Autodesk Inventor part; units mm, degrees
ref_plane "YZ Plane" through (0, 0, 0) normal (1, 0, 0) x (0, 1, 0)
ref_plane "XZ Plane" through (0, 0, 0) normal (0, 1, 0) x (-1, 0, 0)
ref_plane "XY Plane" through (0, 0, 0) normal (0, 0, 1) x (1, 0, 0)
sketch "Sketch1" plane through (0, 0, 0) normal (0, 0, 1) x (1, 0, 0)
  line L0 (3.175, 0) -> (3.175, 3.175)
  line L1 (3.175, 3.175) -> (-3.175, 3.175)
  line L2 (-3.175, 3.175) -> (-3.175, 0)
  line L3 (5.08, 0) -> (5.08, 5.08)
  line L4 (5.08, 5.08) -> (-5.08, 5.08)
  line L5 (-5.08, 5.08) -> (-5.08, 0)
  line L6 (-5.08, 0) -> (-3.175, 0)
  line L7 (3.175, 0) -> (5.08, 0)
  point P0 (0, 0)
  dimension "d0" = 10.16
  dimension "d1" = 5.08
extrude "Extrusion1" add sketch "Sketch1" along normal blind 139.7
sketch "Sketch2" plane through (-5.08, 5.08, 0) normal (0, 1, 0) x (1, 0, 0)
  circle A0 centre (5.08, -6.35) radius 1.985
  circle A1 centre (5.08, -133.35) radius 1.985
  circle A2 centre (5.08, -69.85) radius 1.985
  point P0 (5.08, 0)
  dimension "d4" = 3.97
  dimension "d5" = 3.97
  dimension "d10" = 3.97
extrude "Extrusion2" cut sketch "Sketch2" against normal blind 139.7
sketch "Sketch3" plane through (-5.08, 5.08, 0) normal (0, 1, 0) x (1, 0, 0)
  circle A0 centre (5.08, -6.35) radius 1.985
  circle A1 centre (5.08, -133.35) radius 1.985
  circle A2 centre (5.08, -133.35) radius 5.08
  line L0 (0, 0) -> (0, -139.7)
  circle A3 centre (5.08, -6.35) radius 5.08
  circle A4 centre (5.08, -69.85) radius 1.985
  circle A5 centre (5.08, -69.85) radius 5.08
  point P0 (5.08, 0)
extrude "Extrusion3" add sketch "Sketch3" along normal blind 6.35
properties part number "arm_xbrace_jig"
Geometry check sheet. Reference: the model listing, model coordinates, mm. A direction names the side the tool comes from. Give positions to 0.01 mm unless a question says otherwise; leave off trailing zeros. Write each loop counter-clockwise with the first axis right and the second up, starting at its lowest first coordinate (ties: lowest second). Pieces come first, ordered by that corner, then holes.
1) Release check for a two-part mould opening along Z. For faces 6 (the face through (0, 4, 0)), 7 (the face through (3.175, 2, 69)), 8 (the face through (-1.1, 8.21, 1.39)) record: released by +Z, released by -Z, zero draft, split by the parting line, or undercut.
Values follow:
face 6: released by -Z
face 7: zero draft
face 8: undercut
2) Cross-section at A-A (y = 1.25). Record the boundary of the cut face in (x, z) (3 decimals), plus the area to 3 significant figures.
Values follow:
outline: (-5.08, 0) - (-3.175, 0) - (-3.175, 139.7) - (-5.08, 139.7) - close; (3.175, 0) - (5.08, 0) - (5.08, 139.7) - (3.175, 139.7) - close
area: 532 mm2
3) Cross-section at B-B (x = 0). Record the boundary of the cut face in (y, z) (3 decimals), plus the area to 3 significant figures.
Values follow:
outline: (3.175, 0) - (5.08, 0) - (5.08, 1.27) - (11.43, 1.27) - (11.43, 4.365) - (3.175, 4.365) - close; (3.175, 8.335) - (11.43, 8.335) - (11.43, 11.43) - (5.08, 11.43) - (5.08, 64.77) - (11.43, 64.77) - (11.43, 67.865) - (3.175, 67.865) - close; (3.175, 71.835) - (11.43, 71.835) - (11.43, 74.93) - (5.08, 74.93) - (5.08, 128.27) - (11.43, 128.27) - (11.43, 131.365) - (3.175, 131.365) - close; (3.175, 135.335) - (11.43, 135.335) - (11.43, 138.43) - (5.08, 138.43) - (5.08, 139.7) - (3.175, 139.7) - close
area: 361 mm2
4) Set-up check for faces 1 (the face through (-0.258, 7.36, 4.382)), 2 (the face through (-1.1, 8.21, 64.89)), 3 (the face through (2.2, 11.43, 69.8)), 4 (the face through (0, 5.08, 1)), 5 (the face through (-2, 3.175, 69)): record each of +Z, -Z, +X, -X, +Y, -Y from which the full face is reachable in a straight line by a thin tool's end or side.
Values follow:
face 1: +Y, -Y
face 2: +Y
face 3: +Z, -Z, +X, -X, +Y
face 4: -Z, +Y
face 5: +Z, -Z, -Y
5) Cross-section at D-D (z = 116). Record the boundary of the cut face in (x, y) (3 decimals).
Values follow:
outline: (-5.08, 0) - (-3.175, 0) - (-3.175, 3.175) - (3.175, 3.175) - (3.175, 0) - (5.08, 0) - (5.08, 5.08) - (-5.08, 5.08) - close
6) Go/stop test with flat-tipped pins: pin 1 Ø3 at (x, z) = (0, 103) entering from -Y (3 decimals); pin 2 Ø2.5 at (x, z) = (0, 69.85) entering from -Y; pin 3 Ø5 at (x, z) = (1, 85.5) entering from +Y. Record where each tip stops, or that it passes through.
Values follow:
pin 1: stops at y = 3.175
pin 2: passes through
pin 3: stops at y = 5.08
7) Thickness scan on line 1 (Z direction, x = 0, y = 8.75) (3 decimals); line 2 (X direction, y = 9.5, z = 69.85) (3 decimals); line 3 (Z direction, x = 1, y = 8.5). Record the ranges inside material, lowest first.
Values follow:
line 1: z = 1.27 to 4.365, 8.335 to 11.43, 64.77 to 67.865, 71.835 to 74.93, 128.27 to 131.365, 135.335 to 138.43
line 2: x = -5.08 to -1.985, 1.985 to 5.08
line 3: z = 1.37 to 4.64, 8.06 to 11.33, 64.87 to 68.14, 71.56 to 74.83, 128.37 to 131.64, 135.06 to 138.33
8) Cross-section at C-C (y = 9.5). Record the boundary of the cut face in (x, z) (3 decimals), plus the area to 3 significant figures.
Values follow:
outline: circle Ø10.16 at (0, 6.35); circle Ø10.16 at (0, 69.85); circle Ø10.16 at (0, 133.35); hole circle Ø3.97 at (0, 6.35); hole circle Ø3.97 at (0, 69.85); hole circle Ø3.97 at (0, 133.35)
area: 206 mm2
